Input: dimensioned drawing with shaded views. Units: mm. Origin: part minimum x, y, z. Round coordinates to 2 decimals unless told otherwise and drop trailing zeros. Loops run counter-clockwise (first coordinate to the right, second up) from the corner with the lowest first, then second, coordinate; pieces in that order, holes last.
1) Ray query, line 1 along Y through (x, z) = (27.5, 3.5); line 2 along Y through (x, z) = (27.5, 0.95); line 3 along X through (y, z) = (36.5, 2.5). Return the intervals inside material, ascending.
2) First-contact query: pin 1 (4 mm diameter, centred on x = 43.5, z = 5.5, fed in from -Y); pin 2 (1 mm diameter, centred on x = 32.5, z = 7.5, fed in from +Y); pin 3 (4 mm diameter, centred on x = 23, z = 4.5, fed in from -Y). Flat tips, straight axial feed; report the tip coordinate or a pass-through.
3) Section C-C, the plane z = 6. Return loops of the section in (x, y).
4) Draft query along Y for the marked faces 1, 2, 3 and 4. Return one class per face: pulls with the +Y half, pulls with the -Y half, needs draft (parallel to the pull), parting line crosses it, or undercut.
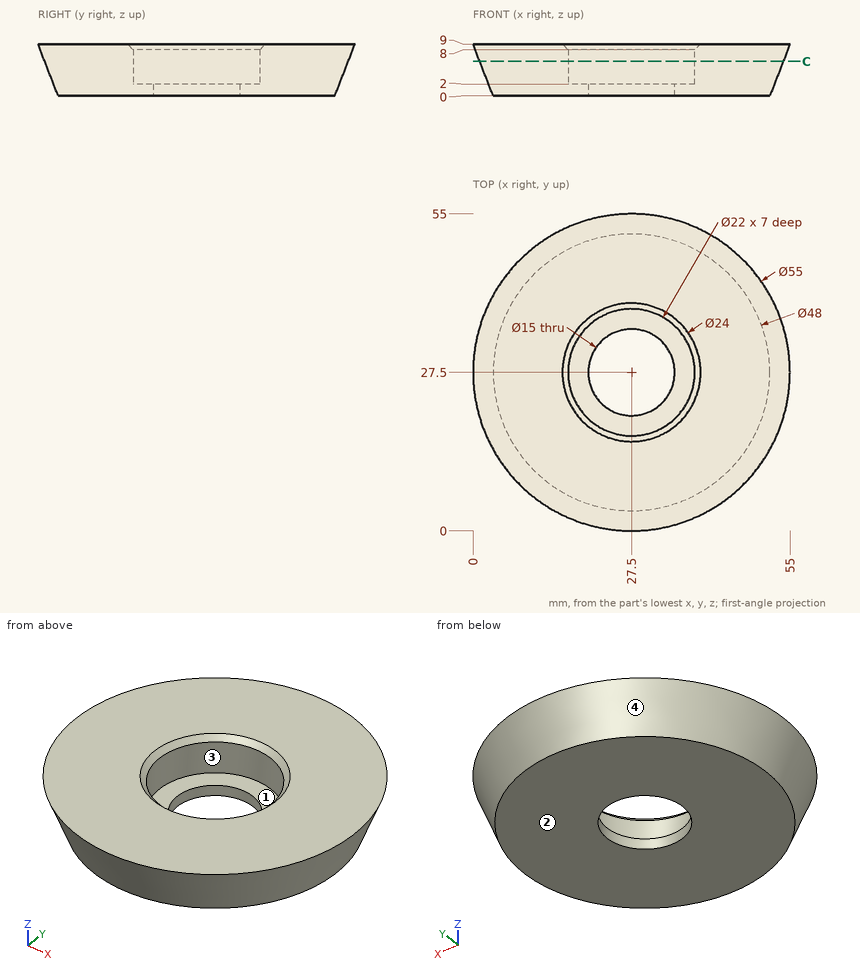
Final values:
1. line 1: y = 2.14 to 16.5, 38.5 to 52.86
1. line 2: y = 3.13 to 20, 35 to 51.87
1. line 3: x = 4.21 to 21.18, 33.82 to 50.79
2. pin 1: stops at y = 5.13
2. pin 2: stops at y = 54.17
2. pin 3: stops at y = 1.3
3. outline: circle Ø52.67 at (27.5, 27.5); hole circle Ø22 at (27.5, 27.5)
4. face 1: undercut
4. face 2: needs draft
4. face 3: undercut
4. face 4: parting line crosses it
